Geometry check sheet. Reference: the model listing, model coordinates, mm. Face numbers are marked on the shaded views. A direction names the side the tool comes from. Give positions to 0.01 mm unless a question says otherwise; leave off trailing zeros. Loops run counter-clockwise (first coordinate to the right, second up) from the corner with the lowest first, then second, coordinate; pieces in that order, holes last. Notation, with made-up numbers: (13.5, 20) -> (50.5, 20) arc R22 ccw to (50.5, 44) -> close; hole circle Ø10 at (-19.5, 15). An arc over 180 degrees is marked (long way). One line per question, with ' | ' between items.
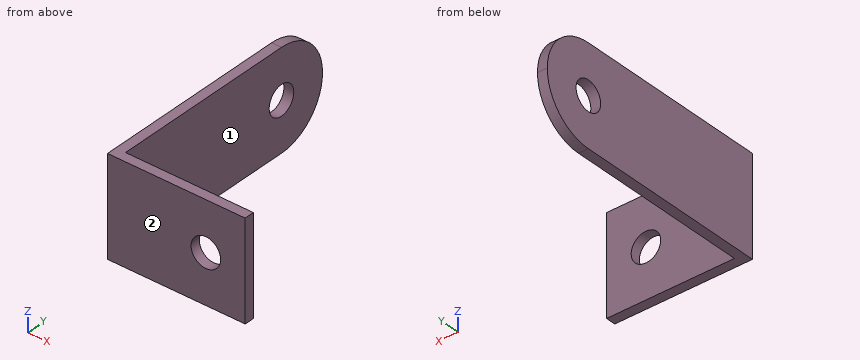
from build123d import *

# Parameters (mm, degrees)
BOSS_EXTRUDE1_DEPTH = 10
FILLET1_R           = 5
SKETCH2_R           = 1.5
CUT_EXTRUDE1_DEPTH  = 30.899832775
SKETCH3_R           = 1.5
CUT_EXTRUDE2_DEPTH  = 30.52964612


with BuildPart() as part:
    # Sketch1 → Boss-Extrude1 (new body)
    with BuildSketch(Plane.XY):
        Polygon((0, 0), (0, 25), (1, 25), (1, 1), (14, 1), (14, 0), align=None)
    extrude(amount=BOSS_EXTRUDE1_DEPTH)

    # Fillet1
    fillet1_edges = [part.edges().sort_by_distance(p)[0] for p in [
        (0.5, 25, 0),
        (0.5, 25, 10),
    ]]
    fillet(fillet1_edges, radius=FILLET1_R - 0.0001)  # a hair under: the kernel refuses the full size

    # Sketch2 → Cut-Extrude1 (cut, through all)
    with BuildSketch(Plane(origin=(1, 0, 0), x_dir=(0, 0, -1), z_dir=(1, 0, 0))):
        with Locations(Location((-5, 20, 0), (0, 0, 90))):
            Circle(SKETCH2_R)
    extrude(amount=-CUT_EXTRUDE1_DEPTH, mode=Mode.SUBTRACT)

    # Sketch3 → Cut-Extrude2 (cut, through all)
    with BuildSketch(Plane(origin=(0, 1, 0), x_dir=(1, 0, 0), z_dir=(0, 1, 0))):
        with Locations(Location((10, -5, 0), (0, 0, 180))):
            Circle(SKETCH3_R)
    extrude(amount=-CUT_EXTRUDE2_DEPTH, mode=Mode.SUBTRACT)


solid = part.part
Item 1: Scan lines: probe 1 along Z at (x, y) = (10, 0.4); probe 2 along Y at (x, z) = (5.5, 3). Record each from-to range of solid material in increasing order.
Result:
probe 1: 0 to 3.5, 6.5 to 10 | probe 2: 0 to 1
Item 2: Sectioned sample at C-C (y = 6.75). Record the cut outline in (x, z), plus the area to 3 significant figures.
Result:
outline: (0, 0) -> (1, 0) -> (1, 10) -> (0, 10) -> close | area: 10.0 mm2
Item 3: Depth check by flat-ended pin: pin 1 Ø3 at (y, z) = (4.5, 9) entering from +X; pin 2 Ø4 at (x, z) = (8.5, 6) entering from +Y. Enter the tip coordinate at first touch or a pass-through.
Result:
pin 1: x = 1 | pin 2: y = 1
Item 4: Sectioned sample at B-B (z = 5.25). Record the cut outline in (x, y).
Result:
outline: (0, 0) -> (8.52, 0) -> (8.52, 1) -> (1, 1) -> (1, 18.52) -> (0, 18.52) -> close; (0, 21.48) -> (1, 21.48) -> (1, 24.99) -> (0, 24.99) -> close; (11.48, 0) -> (14, 0) -> (14, 1) -> (11.48, 1) -> close
Item 5: Set-up check for the marked faces 1 and 2: record each of +Z, -Z, +X, -X, +Y, -Y from which the full face is reachable in a straight line by a thin tool's end or side.
Result:
face 1: +Z, -Z, +X, +Y | face 2: +Z, -Z, +X, -X, -Y
Item 6: Sectioned sample at D-D (z = 7.5). Record the cut outline in (x, y).
Result:
outline: (0, 0) -> (14, 0) -> (14, 1) -> (1, 1) -> (1, 24.33) -> (0, 24.33) -> close
Item 7: Sectioned sample at A-A (x = 10). Record the cut outline in (y, z), plus the area to 3 significant figures.
Result:
outline: (0, 0) -> (1, 0) -> (1, 3.5) -> (0, 3.5) -> close; (0, 6.5) -> (1, 6.5) -> (1, 10) -> (0, 10) -> close | area: 7.00 mm2
